```python
from build123d import *

# Parameters (mm, degrees)
F2_R     = 7.465
F2_R_2   = 7.4
F3_DEPTH = 51.7
F4_R     = 1.720525
F5_DEPTH = 2
F6_R     = 0.31391
F7_DEPTH = 54.198547


with BuildPart() as f1:
    # F0 (on Right) → F1 (revolve)
    with BuildSketch(Plane.YZ):
        Polygon((-4.497547, 0), (0, 0), (0, 6.62), (-0.5, 7.465), (-2.890516, 7.465), (-2.890516, 6.62), (-3.790516, 6.62), (-4.497547, 7.465), align=None)
    revolve(axis=Axis((0, -2.248773, 0), (0, 1, 0)))

    # F2 (on face) → F3 (join)
    with BuildSketch(Plane.XZ.offset(4.497547)):
        Circle(F2_R)
        Circle(F2_R_2, mode=Mode.SUBTRACT)
    extrude(amount=F3_DEPTH)

    # F4 (on face) → F5 (cut)
    with BuildSketch(Plane(origin=(0, 0, 0), x_dir=(-1, 0, 0), z_dir=(0, 1, 0))):
        Circle(F4_R)
    extrude(amount=-F5_DEPTH, mode=Mode.SUBTRACT)

    # F6 (on face) → F7 (cut, through all)
    with BuildSketch(Plane(origin=(0, -2, 0), x_dir=(-1, 0, 0), z_dir=(0, 1, 0))):
        Circle(F6_R)
    extrude(amount=-F7_DEPTH, mode=Mode.SUBTRACT)


solid = f1.part
```
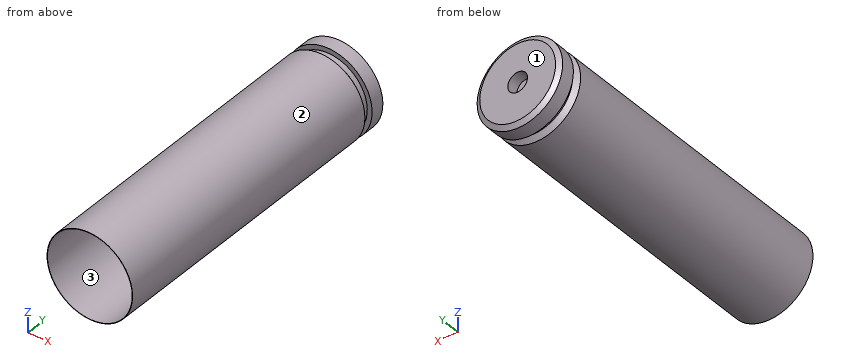
Design review of the part built by this model. Coordinates are the model's own, in mm. Face numbers are marked on the shaded views. Round coordinates to 2 decimals unless told otherwise and drop trailing zeros. Write each loop counter-clockwise with the first axis right and the second up, starting at its lowest first coordinate (ties: lowest second). Pieces come first, ordered by that corner, then holes. Notation, with made-up numbers: (-24, 40.25) -> (21, 40.25) arc R20 cw to (21, 67.25) -> close; hole circle Ø2 at (46.25, -20.75). An arc over 180 degrees is marked (long way). Answer in a Markdown table with one row per item.
Q1. To check wall thickness, follow L1, parallel to Y at x = 3.5, z = -5; L2, parallel to X at y = -4, z = -2. State the ranges of each line that lie inside material, in increasing order. Write a range as [from, to].
The answers:
| item | result |
|---|---|
| L1 | [-4.5, 0] |
| L2 | [-6.57, 6.57] |
Q2. Clearance check with flat-ended pins moving along their axes: pin 1 Ø3 at (y, z) = (-12.5, -1.5) entering from -X (3 decimals); pin 2 Ø3 at (x, y) = (-5.5, -21) entering from +Z; pin 3 Ø7.5 at (x, z) = (-3, -1.5) entering from -Y; pin 4 Ø1 at (x, y) = (2, -13.5) entering from +Z. State where each tip first meets the part, or that it passes through.
The answers:
| item | result |
|---|---|
| pin 1 | x = -7.465 |
| pin 2 | z = 6.3 |
| pin 3 | y = -4.5 |
| pin 4 | z = 7.31 |
Q3. Take a section at A-A, the plane y = -14. State the section outline as (x, z) points (3 decimals).
The answers:
| item | result |
|---|---|
| outline | circle Ø14.93 at (0, 0); hole circle Ø14.8 at (0, 0) |
Q4. Draft analysis for pull direction X (two halves, no side actions). For the marked faces 1, 2 and 3, state which applies: +X half, -X half, draft (parallel to the pull), parting line (faces both ways), or undercut.
The answers:
| item | result |
|---|---|
| face 1 | draft |
| face 2 | parting line |
| face 3 | undercut |
